Work out the finished part from the listing and answer in its coordinate system (mm). A direction names the side the tool comes from. Coordinates: 2 decimals unless noted, no trailing zeros. Order: outer loops, then holes, each group sorted by start corner. A loop starts at its lowest first (then second) coordinate and runs counter-clockwise, first axis right, second up. Notation, with made-up numbers: M 20.25,85.5 L 76.25,85.5 A19 cw 76.25,99.5 Z; hole C 52,-9.75 d9. An arc over 180 degrees is marked long. Answer in a Markdown table with one row per item. Add a question column.
Item 1: Consider line 1 (X direction, y = -49.5, z = 6.75); line 2 (Z direction, x = 31.5, y = 38); line 3 (X direction, y = -48.5, z = 22.5). Determine where each line is inside the solid, lowest interval first. Write a range as from..to.
Item 2: The mould has two halves that part along Y. Classify faces 3 (the face through (18, -78, 29.5)), 4 (the face through (-58.23, 53.39, 24.57)), 5 (the face through (43.545, 68.3, 16.065)): released by +Y, released by -Y, zero draft, split by the parting line, or undercut.
Item 3: The part is cut by section D-D (z = 7.75). Write down the section's boundary in (x, y).
Item 4: The part is cut by section B-B (x = 0). Write down the section's boundary in (y, z), then the cut area to 3 significant figures.
Item 5: Which of the six approach directions +Z, -Z, +X, -X, +Y, -Y give full straight-line access (tool end or side, diameter ignored) to faces 1 (the face through (5.19, -9.98, 1.27)), 2 (the face through (-61.105, -46.853, 10.881))?
Item 6: The part is cut by section C-C (z = 25.5). Write down the section's boundary in (x, y), then the cut area to 3 significant figures.
Item 7: Flat-ended cylindrical pins translate along their axes: pin 1 Ø6 at (x, z) = (-43, 12) entering from +Y; pin 2 Ø5 at (x, y) = (-38, 34) entering from +Z; pin 3 Ø2 at (y, z) = (51.5, 12.5) entering from +X; pin 4 Ø4 at (x, y) = (-8.72, -15.11) entering from -Z. Find the tip coordinate at first contact, or state that the pin passes through.
Item 8: The part is cut by section A-A (y = 0). Write down the section's boundary in (x, z), then the cut area to 3 significant figures.
from build123d import *

# Parameters (mm, degrees)
SKETCH1_R           = 81
BOSS_EXTRUDE1_DEPTH = 2.5
SKETCH2_R           = 11.25
CUT_EXTRUDE1_DEPTH  = 3.5
SKETCH3_R           = 2.6
CUT_EXTRUDE2_DEPTH  = 3.5
SKETCH4_R           = 81
SKETCH4_R_2         = 77
BOSS_EXTRUDE2_DEPTH = 27
SKETCH5_R           = 79
CUT_EXTRUDE3_DEPTH  = 10
FILLET1_R           = 3


with BuildPart() as part:
    # Sketch1 → Boss-Extrude1 (new body)
    with BuildSketch(Plane.XY):
        Circle(SKETCH1_R)
    extrude(amount=BOSS_EXTRUDE1_DEPTH)

    # Sketch2 → Cut-Extrude1 (cut, through all)
    with BuildSketch(Plane.XY.offset(2.5)):
        Circle(SKETCH2_R)
    extrude(amount=-CUT_EXTRUDE1_DEPTH, mode=Mode.SUBTRACT)

    # Sketch3 → Cut-Extrude2 (cut, through all)
    with BuildSketch(Plane.XY.offset(2.5)):
        with Locations((17.45, 0)):
            Circle(SKETCH3_R)
        with Locations((-8.725, 15.112143296)):
            Circle(SKETCH3_R)
        with Locations((-8.725, -15.112143296)):
            Circle(SKETCH3_R)
    extrude(amount=-CUT_EXTRUDE2_DEPTH, mode=Mode.SUBTRACT)

    # Sketch4 → Boss-Extrude2 (add)
    with BuildSketch(Plane.XY.offset(2.5)):
        Circle(SKETCH4_R)
        Circle(SKETCH4_R_2, mode=Mode.SUBTRACT)
    extrude(amount=BOSS_EXTRUDE2_DEPTH)

    # Sketch5 → Cut-Extrude3 (cut)
    with BuildSketch(Plane.XY.offset(29.5)):
        Circle(SKETCH5_R)
    extrude(amount=-CUT_EXTRUDE3_DEPTH, mode=Mode.SUBTRACT)

    # Fillet1
    fillet1_edges = [part.edges().sort_by_distance(p)[0] for p in [
        (-81, 0, 0),
    ]]
    fillet(fillet1_edges, radius=FILLET1_R)


solid = part.part
Reply:
| question | item | result |
|---|---|---|
| 1 | line 1 | x = -64.12..-58.98, 58.98..64.12 |
| 1 | line 2 | z = 0..2.5 |
| 1 | line 3 | x = -64.87..-62.36, 62.36..64.87 |
| 2 | face 3 | zero draft |
| 2 | face 4 | undercut |
| 2 | face 5 | split by the parting line |
| 3 | outline | C 0,0 d162; hole C 0,0 d154 |
| 4 | outline | M -81,3 A3 ccw -78,0 L -11.25,0 L -11.25,2.5 L -77,2.5 L -77,19.5 L -79,19.5 L -79,29.5 L -81,29.5 Z; M 11.25,0 L 78,0 A3 ccw 81,3 L 81,29.5 L 79,29.5 L 79,19.5 L 77,19.5 L 77,2.5 L 11.25,2.5 Z |
| 4 | area | 521 mm2 |
| 5 | face 1 | +Z, -Z |
| 5 | face 2 | +Z |
| 6 | outline | C 0,0 d162; hole C 0,0 d158 |
| 6 | area | 1,010 mm2 |
| 7 | pin 1 | stops at y = 70.43 |
| 7 | pin 2 | stops at z = 2.5 |
| 7 | pin 3 | stops at x = 63.33 |
| 7 | pin 4 | passes through |
| 8 | outline | M -81,3 A3 ccw -78,0 L -11.25,0 L -11.25,2.5 L -77,2.5 L -77,19.5 L -79,19.5 L -79,29.5 L -81,29.5 Z; M 11.25,0 L 14.85,0 L 14.85,2.5 L 11.25,2.5 Z; M 20.05,0 L 78,0 A3 ccw 81,3 L 81,29.5 L 79,29.5 L 79,19.5 L 77,19.5 L 77,2.5 L 20.05,2.5 Z |
| 8 | area | 508 mm2 |
